Check sheet for the modelled part. Datum: model origin and axes. Units: mm. Face numbers are marked on the shaded views. Give positions to 0.01 mm unless a question says otherwise; leave off trailing zeros. Order: outer loops, then holes, each group sorted by start corner. A loop starts at its lowest first (then second) coordinate and runs counter-clockwise, first axis right, second up. Notation, with made-up numbers: M 43,-6.75 L 91,-6.75 A21 ccw 91,-1.75 Z; hole C -2,62.5 d6. An arc over 180 degrees is marked long. Answer in a Markdown table with one row per item. Add a question column.
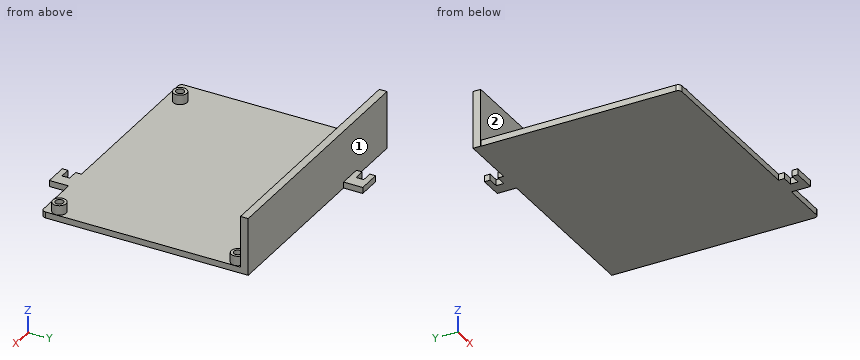
from build123d import *

# Parameters (mm, degrees)
SKETCH1_R             = 3.5
SKETCH1_R_2           = 2.1
BOSS_EXTRUDE1_DEPTH   = 5
BOSS_EXTRUDE1_2_DEPTH = 5
BOSS_EXTRUDE1_3_DEPTH = 5
BOSS_EXTRUDE1_4_DEPTH = 5
SKETCH2_W             = 129.83
SKETCH2_H             = 103.668
BOSS_EXTRUDE2_DEPTH   = 3.175
SKETCH3_W             = 129.972581898
SKETCH3_H             = 4
BOSS_EXTRUDE3_DEPTH   = 30
FILLET1_R             = 2
BOSS_EXTRUDE4_DEPTH   = 3.175


with BuildPart() as part:
    # Sketch1 → Boss-Extrude1 (new body)
    with BuildSketch(Plane(origin=(0, 0, -78.144797939), x_dir=(-1, 0, 0), z_dir=(0, 0, -1))):
        with Locations((153.123589598, -2.351422522)):
            Circle(SKETCH1_R)
        with Locations((153.123589598, -2.351422522)):
            Circle(SKETCH1_R_2, mode=Mode.SUBTRACT)
    extrude(amount=BOSS_EXTRUDE1_DEPTH)



with BuildPart() as body_2:
    # Sketch1 → Boss-Extrude1 2 (new body)
    with BuildSketch(Plane(origin=(0, 0, -78.144797939), x_dir=(-1, 0, 0), z_dir=(0, 0, -1))):
        with Locations((266.153589598, -2.351422522)):
            Circle(SKETCH1_R)
        with Locations((266.153589598, -2.351422522)):
            Circle(SKETCH1_R_2, mode=Mode.SUBTRACT)
    extrude(amount=BOSS_EXTRUDE1_2_DEPTH)


with BuildPart() as body_3:
    # Sketch1 → Boss-Extrude1 3 (new body)
    with BuildSketch(Plane(origin=(0, 0, -78.144797939), x_dir=(-1, 0, 0), z_dir=(0, 0, -1))):
        with Locations((153.123589598, -95.315422522)):
            Circle(SKETCH1_R)
        with Locations((153.123589598, -95.315422522)):
            Circle(SKETCH1_R_2, mode=Mode.SUBTRACT)
    extrude(amount=BOSS_EXTRUDE1_3_DEPTH)


with BuildPart() as body_4:
    # Sketch1 → Boss-Extrude1 4 (new body)
    with BuildSketch(Plane(origin=(0, 0, -78.144797939), x_dir=(-1, 0, 0), z_dir=(0, 0, -1))):
        with Locations((266.153589598, -95.315422522)):
            Circle(SKETCH1_R)
        with Locations((266.153589598, -95.315422522)):
            Circle(SKETCH1_R_2, mode=Mode.SUBTRACT)
    extrude(amount=BOSS_EXTRUDE1_4_DEPTH)


with BuildPart() as part_1:
    add(part.part)

    add(body_2.part)  # Boss-Extrude2 merges body 2

    add(body_3.part)  # Boss-Extrude2 merges body 3

    add(body_4.part)  # Boss-Extrude2 merges body 4
    # Sketch2 → Boss-Extrude2 (add)
    with BuildSketch(Plane(origin=(0, 0, -83.144797939), x_dir=(-1, 0, 0), z_dir=(0, 0, -1))):
        with Locations((214.464589598, -50.865422522)):
            Rectangle(SKETCH2_W, SKETCH2_H)
    extrude(amount=BOSS_EXTRUDE2_DEPTH)

    # Sketch3 → Boss-Extrude3 (add)
    with BuildSketch(Plane(origin=(0, 0, -86.319797939), x_dir=(-1, 0, 0), z_dir=(0, 0, -1))):
        with Locations((214.535880547, 2.968577478)):
            Rectangle(SKETCH3_W, SKETCH3_H)
    extrude(amount=-BOSS_EXTRUDE3_DEPTH)

    # Fillet1
    fillet1_edges = [part_1.edges().sort_by_distance(p)[0] for p in [
        (-279.379589598, -102.699422522, -84.732297939),
        (-149.549589598, -102.699422522, -84.732297939),
    ]]
    fillet(fillet1_edges, radius=FILLET1_R)

    # Sketch4 → Boss-Extrude4 (add)
    with BuildSketch(Plane(origin=(0, 0, -86.319797939), x_dir=(-1, 0, 0), z_dir=(0, 0, -1))):
        Polygon((238.851684859, 14.968577478), (238.851684859, 4.968577478), (250.851684859, 4.968577478), (250.851684859, 7.968577478), (245.201684859, 7.968577478), (245.201684859, 11.968577478), (250.851684859, 11.968577478), (250.851684859, 14.968577478), align=None)
        Polygon((187.002486437, -102.699422522), (175.002486437, -102.699422522), (175.002486437, -112.699422522), (187.002486437, -112.699422522), (187.002486437, -109.699422522), (181.352486437, -109.699422522), (181.352486437, -105.699422522), (187.002486437, -105.699422522), align=None)
    extrude(amount=-BOSS_EXTRUDE4_DEPTH)


solid = part_1.part
Q1. Cross-section at B-B (y = -87). Record the boundary of the cut face in (x, z), and give its area (3 significant figures).
Q2. Cross-section at D-D (z = -76.5). Record the boundary of the cut face in (x, y).
Q3. Thickness scan on probe 1 along Y at (x, z) = (-157.5, -58.5); probe 2 along Z at (x, y) = (-247, -76); probe 3 along Y at (x, z) = (-219, -83.25). Record the ranges inside material, lowest first.
Q4. Go/stop test with flat-tipped pins: pin 1 (3.5 mm diameter, centred on x = -153.12, y = -95.32, fed in from +Z); pin 2 (1.6 mm diameter, centred on x = -162.5, z = -84.5, fed in from -Y); pin 3 (1 mm diameter, centred on x = -183.5, z = -84, fed in from +Y). Record where each tip stops, or that it passes through.
Q5. Cross-section at C-C (x = -160). Record the boundary of the cut face in (y, z), and give its area (3 significant figures).
Q6. Cross-section at A-A (x = -248). Record the boundary of the cut face in (y, z).
Q7. Draft check along X on the marked faces 1 and 2. Enter one of: pulls with the +X half, pulls with the -X half, needs draft (parallel to the pull), parting line crosses it, or undercut.
Values follow:
| question | item | result |
|---|---|---|
| 1 | outline | M -279.38,-86.32 L -149.55,-86.32 L -149.55,-83.14 L -279.38,-83.14 Z |
| 1 | area | 412 mm² |
| 2 | outline | M -279.52,0.97 L -149.55,0.97 L -149.55,4.97 L -279.52,4.97 Z |
| 3 | probe 1 | 0.97 to 4.97 |
| 3 | probe 2 | -86.32 to -83.14 |
| 3 | probe 3 | -102.7 to 4.97 |
| 4 | pin 1 | z = -83.14 |
| 4 | pin 2 | y = -102.7 |
| 4 | pin 3 | y = 4.97 |
| 5 | outline | M -102.7,-86.32 L 4.97,-86.32 L 4.97,-56.32 L 0.97,-56.32 L 0.97,-83.14 L -102.7,-83.14 Z |
| 5 | area | 449 mm² |
| 6 | outline | M -102.7,-86.32 L 7.97,-86.32 L 7.97,-83.14 L 4.97,-83.14 L 4.97,-56.32 L 0.97,-56.32 L 0.97,-83.14 L -102.7,-83.14 Z; M 11.97,-86.32 L 14.97,-86.32 L 14.97,-83.14 L 11.97,-83.14 Z |
| 7 | face 1 | needs draft |
| 7 | face 2 | undercut |
